Design review of the part built by this model. Coordinates are the model's own, in mm. Round coordinates to 2 decimals unless told otherwise and drop trailing zeros. Loops run counter-clockwise (first coordinate to the right, second up) from the corner with the lowest first, then second, coordinate; pieces in that order, holes last. Notation, with made-up numbers: (-6.75, -15.75) -> (33.25, -15.75) arc R20 cw to (33.25, 10.25) -> close; hole circle Ø5 at (68.5, -11). An arc over 180 degrees is marked (long way). Answer as CSV lines item,"result". Start each with the question number.
(1) Take a section at D-D, the plane y = -3.5. Write out the cut boundary in (x, z), and give its area (3 significant figures).
(2) To check wall thickness, follow line 1 (Y direction, x = 0, z = 0.6); line 2 (X direction, y = 1, z = 0.1); line 3 (X direction, y = -0.5, z = 0.3). State the ranges of each line that lie inside material, in increasing order. Write a range as from..to.
(3) For P1, Ø3, axis at x = 0.5, y = 1, coming from the +Z side, flat-tipped, find the tip position at first contact; note if it passes through.
(4) Take a section at C-C, the plane z = -0.35. Write out the cut boundary in (x, y).
(5) Take a section at A-A, the plane x = 0. Write out the cut boundary in (y, z), and give its area (3 significant figures).
(6) Take a section at B-B, the plane y = 0.75. Write out the cut boundary in (x, z).
Autodesk Inventor part; units mm, degrees
ref_plane "YZ Plane" through (0, 0, 0) normal (1, 0, 0) x (0, 1, 0)
ref_plane "XZ Plane" through (0, 0, 0) normal (0, 1, 0) x (-1, 0, 0)
ref_plane "XY Plane" through (0, 0, 0) normal (0, 0, 1) x (1, 0, 0)
sketch "Sketch1" plane through (0, 0, 0) normal (0, 0, 1) x (1, 0, 0)
  line L0 (2.8868, 5) -> (5.7735, 0)
  line L1 (5.7735, 0) -> (2.8868, -5)
  line L2 (2.8868, -5) -> (-2.8868, -5)
  line L3 (-2.8868, -5) -> (-5.7735, 0)
  line L4 (-5.7735, 0) -> (-2.8868, 5)
  line L5 (-2.8868, 5) -> (2.8868, 5)
  point P0 (0, 0)
  point P1 (0, 0)
  dimension "d0" = 10
extrude "Extrusion1" add sketch "Sketch1" along normal mid plane 2.2
sketch "Sketch2" plane through (0, 0, 1.1) normal (0, 0, 1) x (1, 0, 0)
  circle A0 centre (0, 0) radius 3.1
  dimension "d3" = 6.2
extrude "Extrusion2" cut sketch "Sketch2" against normal through all
sketch "Sketch3" plane through (0, 0, 0) normal (1, 0, 0) x (0, 1, 0)
  line L0 (3.1, -1.1) -> (3.1, -1.6889)
  line L1 (3.1, -1.1) -> (3.61, -1.3944)
  line L2 (3.61, -1.3944) -> (3.1, -1.6889)
  line L3 (3.1, -1.1) -> (3.61, -1.3944)
  line L4 (3.1, -1.6889) -> (3.1, -1.1)
  point P0 (0, 0)
properties part number "Porca Potenciometro"
The answers:
1,outline,"(-3.75, -1.1) -> (3.75, -1.1) -> (3.75, 1.1) -> (-3.75, 1.1) -> close"
1,area,"16.5 mm²"
2,line 1,"-5..-3.1, 3.1..5"
2,line 2,"-5.2..-2.93, 2.93..5.2"
2,line 3,"-5.48..-3.06, 3.06..5.48"
3,P1,"through"
4,outline,"(-5.77, 0) -> (-2.89, -5) -> (2.89, -5) -> (5.77, 0) -> (2.89, 5) -> (-2.89, 5) -> close; hole circle Ø6.2 at (0, 0)"
5,outline,"(-5, -1.1) -> (-3.1, -1.1) -> (-3.1, 1.1) -> (-5, 1.1) -> close; (3.1, -1.1) -> (5, -1.1) -> (5, 1.1) -> (3.1, 1.1) -> close"
5,area,"8.36 mm²"
6,outline,"(-5.34, -1.1) -> (-3.01, -1.1) -> (-3.01, 1.1) -> (-5.34, 1.1) -> close; (3.01, -1.1) -> (5.34, -1.1) -> (5.34, 1.1) -> (3.01, 1.1) -> close"
